Geometry check sheet. Reference: the model listing, model coordinates, mm. A direction names the side the tool comes from. Coordinates: 2 decimals unless noted, no trailing zeros. Order: outer loops, then holes, each group sorted by start corner. A loop starts at its lowest first (then second) coordinate and runs counter-clockwise, first axis right, second up. Notation, with made-up numbers: (53, -17) - (68, -17) arc R33 ccw to (68, 17) - close; hole circle Ø8 at (42, 19). An arc over 180 degrees is marked (long way). Use CSV: the item, a comma, the result in double quotes. Start each with the question number.
1) Depth check by flat-ended pin: P1, Ø1.8, axis at x = 0, z = 0, coming from the +Y side; P2, Ø3, axis at x = -3, z = -1.5, coming from the +Y side; P3, Ø3, axis at x = 2.5, y = 9, coming from the +Z side; P4, Ø1, axis at y = 10.5, z = 0.5, coming from the -X side. Enter the tip coordinate at first touch or a pass-through.
2) Sectioned sample at A-A, the plane y = 11.5. Record the cut outline in (x, z).
3) Sectioned sample at B-B, the plane z = 4.25. Record the cut outline in (x, y), and give its area (3 significant figures).
4) Tool access check on faces 1 (the flat face through (0, 5, -3.4)), 2 (the cylindrical face through (-3, 12, 0)), 3 (the flat face through (4, 7, 0)). Record the directions out of +Z, -Z, +X, -X, +Y, -Y that give a thin tool (end or side, any length) a straight path to the whole face; none if there is none.
5) Thickness scan on probe 1 along Z at (x, y) = (0, 9.25); probe 2 along Y at (x, z) = (1, 0.25); probe 3 along X at (y, z) = (3.45, 0). Record the ranges inside material, lowest first. Write a range as [from, to].
6) Draft check along Z on faces 4 (the conical face through (-1.506, 3.792, -0.022)), 5 (the cylindrical face through (0, 10, 1)), 6 (the flat face through (2.028, 6.521, 3.448)). Enter one of: released by +Z, released by -Z, zero draft, split by the parting line, or undercut.
Autodesk Inventor part; units mm, degrees
ref_plane "Plano de trabajo1" through (0, 8, 0) normal (0, 1, 0) x (-1, 0, 0)
ref_plane "Plano de trabajo6" through (0, 3.8, 0) normal (0, -1, 0) x (1, 0, 0)
ref_plane "YZ Plane" through (0, 0, 0) normal (1, 0, 0) x (0, 1, 0)
ref_plane "Plano de trabajo1" through (0, 8, 0) normal (0, 1, 0) x (-1, 0, 0)
sketch "Boceto2" plane through (0, 8, 0) normal (0, 1, 0) x (-1, 0, 0)
  line L0 (0, -4.6188) -> (-4, -2.3094)
  line L1 (-4, -2.3094) -> (-4, 2.3094)
  line L2 (-4, 2.3094) -> (0, 4.6188)
  line L3 (0, 4.6188) -> (4, 2.3094)
  line L4 (4, 2.3094) -> (4, -2.3094)
  line L5 (4, -2.3094) -> (0, -4.6188)
  point P0 (0, 0)
  point P1 (0, 0)
  dimension "d2" = 8
extrude "Extrusión1" add sketch "Boceto2" against normal blind 3
sketch "Boceto3" plane through (0, 8, 0) normal (0, 1, 0) x (1, 0, 0)
  circle A0 centre (0, 0) radius 3
  circle A1 centre (0, 0) radius 3
  dimension "d9" = 6
  dimension "d10" = 6
extrude "Extrusión2" add sketch "Boceto3" along normal blind 1
sketch "Boceto4" plane through (0, 9, 0) normal (0, 1, 0) x (1, 0, 0)
  circle A0 centre (0, 0) radius 3
extrude "Extrusión3" add sketch "Boceto4" along normal blind 6.5
sketch "Boceto6" plane through (0, 15.5, 0) normal (0, 1, 0) x (1, 0, 0)
  circle A0 centre (0, 0) radius 1
  dimension "d26" = 2
extrude "Extrusión4" cut sketch "Boceto6" against normal blind 12.25
sketch "Boceto12" plane through (0, 5, 0) normal (0, -1, 0) x (1, 0, 0)
  circle A0 centre (0, 0) radius 1
  line L0 (-1.8028, 3) -> (1.8028, 3)
  arc A1 (1.8028, -3) -> (1.8028, 3) centre (0, 0) ccw
  arc A2 (-1.8028, 3) -> (-1.8028, -3) centre (0, 0) ccw
  line L1 (1.8028, -3) -> (-1.8028, -3)
ref_plane "Plano de trabajo6" through (0, 3.8, 0) normal (0, -1, 0) x (1, 0, 0)
ref_plane "Plano de trabajo5" through (0, 3, 0) normal (0, -1, 0) x (1, 0, 0)
sketch "Boceto13" plane through (0, 3, 0) normal (0, -1, 0) x (1, 0, 0)
  circle A0 centre (0, 0) radius 0.2
  dimension "d44" = 0.4
sketch "Boceto14" plane through (0, 3.8, 0) normal (0, -1, 0) x (1, 0, 0)
  circle A0 centre (0, 0) radius 0.2
  dimension "d45" = 0.4
loft "Solevación2" add profiles "Boceto12", "Boceto13" contours A0 | L0 A1 L1 A2 / all
loft "Solevación3" cut profiles "Boceto14" section 2 edges at (-1, 5, 0)
sketch "Boceto15" plane through (0, 3, 0) normal (0, -1, 0) x (0.9991294, 0, 0.0417196)
  circle A0 centre (0, 0) radius 0.2
  dimension "d54" = 0.4
extrude "Extrusión8" cut sketch "Boceto15" against normal blind 2
properties part number "boquilla 0.4" material "Latón, amarillo claro"
Evaluation:
1,P1,"y = 4.85"
1,P2,"y = 15.5"
1,P3,"z = 3.82"
1,P4,"x = -3"
2,outline,"circle Ø6 at (0, 0); hole circle Ø2 at (0, 0)"
3,outline,"(-0.64, 5) - (0.64, 5) - (0.64, 8) - (-0.64, 8) - close"
3,area,"3.83 mm²"
4,face 1,"-Y"
4,face 2,"+Y"
4,face 3,"+Z, -Z, +X, +Y, -Y"
5,probe 1,"[-3, -1], [1, 3]"
5,probe 2,"[3.5, 15.5]"
5,probe 3,"[-0.94, -0.2], [0.2, 0.94]"
6,face 4,"split by the parting line"
6,face 5,"undercut"
6,face 6,"released by +Z"
